from build123d import *

# Parameters (mm, degrees)
F0_W           = 30
F0_H           = 45
F1_DEPTH       = 4
F3_D           = 2
F3_DEPTH       = 20
F3_TIP         = 0.600860619
F4_W           = 2
F4_H           = 45
F5_DEPTH       = 2
F6_W           = 3
F6_H           = 19
F7_DEPTH       = 0.5
F8_D           = 3
F8_DEPTH       = 6
F8_CBORE_D     = 6
F8_CBORE_DEPTH = 2
F8_TIP         = 0.9012909285


with BuildPart() as f1:
    # F0 (on Top) → F1 (new body)
    with BuildSketch(Plane.XY):
        Rectangle(F0_W, F0_H)
    extrude(amount=F1_DEPTH)

    # F3
    with Locations(Plane(origin=(0, 22.5, 0), x_dir=(-1, 0, 0), z_dir=(0, 1, 0))):
        with Locations((-7, 2), (7, 2)):
            Hole(F3_D / 2, depth=F3_DEPTH)
            with Locations((0, 0, -(F3_DEPTH + F3_TIP / 2))):  # 118° drill point
                Cone(0, F3_D / 2, F3_TIP, mode=Mode.SUBTRACT)

    # F4 (on face) → F5 (join)
    with BuildSketch(Plane.XY.offset(4)):
        with Locations((-14, 0)):
            Rectangle(F4_W, F4_H)
        with Locations((14, 0)):
            Rectangle(F4_W, F4_H)
    extrude(amount=F5_DEPTH)

    # F6 (on face) → F7 (cut)
    with BuildSketch(Plane(origin=(0, 0, 0), x_dir=(1, 0, 0), z_dir=(0, 0, -1))):
        with Locations((0, -13)):
            Rectangle(F6_W, F6_H)
    extrude(amount=-F7_DEPTH, mode=Mode.SUBTRACT)

    # F8
    with Locations(Plane(origin=(0, 0, 0), x_dir=(1, 0, 0), z_dir=(0, 0, -1))):
        with Locations((0, 0)):
            CounterBoreHole(F8_D / 2, F8_CBORE_D / 2, F8_CBORE_DEPTH, depth=F8_DEPTH)
            with Locations((0, 0, -(F8_DEPTH + F8_TIP / 2))):  # 118° drill point
                Cone(0, F8_D / 2, F8_TIP, mode=Mode.SUBTRACT)


solid = f1.part
Model file for the job. Use its own axes, mm. A direction names the side the tool comes from. Give positions to 0.01 mm unless a question says otherwise; leave off trailing zeros. Order: outer loops, then holes, each group sorted by start corner. A loop starts at its lowest first (then second) coordinate and runs counter-clockwise, first axis right, second up. Notation, with made-up numbers: M -9,57.25 L 48,57.25 A19 ccw 48,75.25 Z; hole C 60.25,-18.75 d8. An arc over 180 degrees is marked long. Put each result on its own line as item: value. Start each with the question number.
(1) Drill centre lines: L1, parallel to X at y = 9.75, z = 2; L2, parallel to Y at x = 0, z = 3.2; L3, parallel to Z at x = 7, y = 9. Where is each one in solid material? Low to high. Write a range as [from, to].
(2) Tool access for faces 1 (the face through (-13, 0, 5)), 2 (the face through (6.2, 12.4, 1.4)), 3 (the face through (0, 13, 0.5)): list every direction of +Z, -Z, +X, -X, +Y, -Y with a clear straight run to the whole face (end or side of a thin tool).
(3) Band-saw the part on C-C on y = -7. Give the cut face in (x, z).
(4) Band-saw the part on D-D on y = 1. Give the cut face in (x, z).
(5) Pull direction Z, two halves, no side cores. Call faces 4 (the face through (15, 0, 3)), 5 (the face through (-3, 0, 4)), 6 (the face through (-7, 12, 1)): released by +Z, released by -Z, zero draft, split by the parting line, or undercut.
(6) Pin check, flat tips, straight feed: pin 1 Ø0.9 at (x, y) = (0, 13) entering from -Z; pin 2 Ø1.8 at (x, y) = (0, 0) entering from -Z; pin 3 Ø1.6 at (x, z) = (-7, 2) entering from +Y. Stop position of each tip, or through.
(7) Band-saw the part on A-A on x = 0. Give the cut face in (y, z), then the cut area to 4 significant figures.
(8) Band-saw the part on B-B on y = 9. Give the cut face in (x, z).
Results below:
1. L1: x = [-15, -8], [-6, 6], [8, 15]
1. L2: y = [-22.5, -1.5], [1.5, 22.5]
1. L3: z = [0, 1], [3, 4]
2. face 1: +Z, +Y, -Y
2. face 2: +Y
2. face 3: -Z, +Y
3. outline: M -15,0 L 15,0 L 15,6 L 13,6 L 13,4 L -13,4 L -13,6 L -15,6 Z
4. outline: M -15,0 L -2.83,0 L -2.83,2 L -1.12,2 L -1.12,4 L -13,4 L -13,6 L -15,6 Z; M 1.12,2 L 2.83,2 L 2.83,0 L 15,0 L 15,6 L 13,6 L 13,4 L 1.12,4 Z
5. face 4: zero draft
5. face 5: released by +Z
5. face 6: undercut
6. pin 1: stops at z = 0.5
6. pin 2: passes through
6. pin 3: stops at y = 2.38
7. outline: M -22.5,0 L -3,0 L -3,2 L -1.5,2 L -1.5,4 L -22.5,4 Z; M 1.5,2 L 3,2 L 3,0 L 3.5,0 L 3.5,0.5 L 22.5,0.5 L 22.5,4 L 1.5,4 Z
7. area: 152.5 mm2
8. outline: M -15,0 L -1.5,0 L -1.5,0.5 L 1.5,0.5 L 1.5,0 L 15,0 L 15,6 L 13,6 L 13,4 L -13,4 L -13,6 L -15,6 Z; hole C -7,2 d2; hole C 7,2 d2
